Design review of the part built by this model. Coordinates are the model's own, in mm. Face numbers are marked on the shaded views. A direction names the side the tool comes from. Coordinates: 2 decimals unless noted, no trailing zeros. Loops run counter-clockwise (first coordinate to the right, second up) from the corner with the lowest first, then second, coordinate; pieces in that order, holes last. Notation, with made-up numbers: M -5.75,-33.75 L 7.25,-33.75 A13 cw 7.25,-21.75 Z; hole C -31.5,63.5 d11. An arc over 180 degrees is marked long. Put each result on its own line as item: value. Start each with the question number.
(1) Take a section at D-D, the plane y = 2.5. Give the boundary of the cut face in (x, z), then the cut area to 3 significant figures.
(2) For probe 1 along X at (y, z) = (-5.75, 3.25); probe 2 along X at (y, z) = (-0.75, 0.5); probe 3 along Z at (x, y) = (14.5, 0), list the stretches that pass through material, from the lowest coordinate up. Write a range as [from, to].
(3) Take a section at A-A, the plane x = 20. Count the separate pieces of the cut face and the enclosed holes in it, then the cut area to 3 significant figures.
(4) The part is to be moulded in two halves that separate along Y. For the marked faces 1, 2, 3 and 4, say which applies: +Y half, -Y half, draft (parallel to the pull), parting line (faces both ways), or undercut.
(5) For the marked faces 5, 6 and 7, list the 3-axis set-ups (+Z, -Z, +X, -X, +Y, -Y) from which the entire face can be reached by the end or side of a thin tool; tool diameter is ignored.
(6) Clearance check with flat-ended pins moving along their axes: pin 1 (8 mm diameter, centred on x = 23, y = -1.5, fed in from -Z); pin 2 (2 mm diameter, centred on x = 23, z = 1, fed in from -Y); pin 3 (1.3 mm diameter, centred on x = 14.5, z = 1.5, fed in from -Y); pin 4 (1 mm diameter, centred on x = 0.5, y = -3.5, fed in from +Z). State where each tip first meets the part, or that it passes through.
Autodesk Inventor part; units mm, degrees
ref_plane "YZ Plane" through (0, 0, 0) normal (1, 0, 0) x (0, 1, 0)
ref_plane "XZ Plane" through (0, 0, 0) normal (0, 1, 0) x (-1, 0, 0)
ref_plane "XY Plane" through (0, 0, 0) normal (0, 0, 1) x (1, 0, 0)
sketch "Sketch1" plane through (0, 0, 0) normal (0, 0, 1) x (1, 0, 0)
  line L0 (-21.147, 7.3925) -> (29.653, 7.3925)
  line L1 (29.653, 7.3925) -> (29.653, -5.3075)
  line L2 (29.653, -5.3075) -> (-21.147, -5.3075)
  line L3 (-21.147, -5.3075) -> (-21.147, 7.3925)
  point P0 (0, 0)
  dimension "d0" = 50.8
  dimension "d1" = 12.7
extrude "Extrusion1" add sketch "Sketch1" along normal blind 2.54
sketch "Sketch3" plane through (29.653, -5.3075, 0) normal (1, 0, 0) x (0, 0, -1)
  line L0 (-2.54, 0) -> (-8.89, 0)
  line L1 (-8.89, 0) -> (-8.89, -6.35)
  line L2 (-8.89, -6.35) -> (-2.54, -6.35)
  line L3 (-2.54, -6.35) -> (-2.54, 0)
  point P0 (0, 5.3075)
  dimension "d9" = 6.35
  dimension "d10" = 6.35
extrude "Extrusion2" add sketch "Sketch3" against normal blind 50.8
fillet "Fillet1" radius 3.175 3 edges at (4.253, -5.3075, 8.89) (4.253, -11.6575, 8.89) (4.253, -11.6575, 2.54)
hole "Hole1" at (29.653, -8.4825, 5.715) direction (-1, 0, 0) diameter 5.08 end through all
sketch "Sketch4" plane through (-21.147, -5.3075, 2.54) normal (0, 1, 0) x (1, 0, 0)
  line L0 (50.8, 0) -> (0, 0)
  line L1 (0, 0) -> (0, -3.175)
  line L2 (6.35, 0) -> (12.7, 0)
  line L3 (12.7, 0) -> (12.7, -6.6787)
  line L4 (12.7, -6.6787) -> (6.35, -6.6787)
  line L5 (6.35, -6.6787) -> (6.35, 0)
  line L6 (19.05, 0) -> (25.4, 0)
  line L7 (25.4, 0) -> (25.4, -6.6787)
  line L8 (25.4, -6.6787) -> (19.05, -6.6787)
  line L9 (19.05, -6.6787) -> (19.05, 0)
  line L10 (31.75, 0) -> (38.1, 0)
  line L11 (38.1, 0) -> (38.1, -6.6787)
  line L12 (38.1, -6.6787) -> (31.75, -6.6787)
  line L13 (31.75, -6.6787) -> (31.75, 0)
  point P0 (21.147, 2.54)
  dimension "d23" = 6.35
  dimension "d24" = 6.35
  dimension "d25" = 6.35
  dimension "d26" = 6.35
  dimension "d27" = 6.35
  dimension "d28" = 6.35
extrude "Extrusion3" cut sketch "Sketch4" against normal blind 12.7
hole "Hole2" at (-9.717, 1.0425, 2.54) direction (0, 0, -1) diameter 4.9784 end through all
hole "Hole3" at (18.223, 1.0425, 2.54) direction (0, 0, -1) diameter 4.9784 end through all
hole "Hole4" at (4.253, 1.0425, 2.54) direction (0, 0, -1) diameter 4.9784 end through all
sketch "Sketch5" plane through (29.653, -8.4825, 2.54) normal (0, 0, -1) x (-1, 0, 0)
  line L0 (12.7, 0) -> (12.7, 3.175)
  line L1 (0, 3.175) -> (12.7, 3.175)
  line L2 (0, 3.175) -> (12.7, 3.175)
  line L3 (12.7, 3.175) -> (12.7, 0)
  line L4 (12.7, 0) -> (0, 0)
  line L5 (0, 0) -> (0, 3.175)
  point P0 (29.653, 8.4825)
sketch "Sketch6" plane through (10.603, -8.4825, 2.54) normal (0, 0, -1) x (-1, 0, 0)
  line L0 (0, 3.175) -> (0, 0)
  line L1 (6.35, 0) -> (0, 0)
  line L2 (0, 3.175) -> (6.35, 3.175)
  line L3 (6.35, 3.175) -> (6.35, 0)
  line L4 (6.35, 0) -> (0, 0)
  line L5 (0, 0) -> (0, 3.175)
  point P0 (10.603, 8.4825)
sketch "Sketch7" plane through (-2.097, -8.4825, 2.54) normal (0, 0, -1) x (-1, 0, 0)
  line L0 (0, 3.175) -> (0, 0)
  line L1 (6.35, 0) -> (0, 0)
  line L2 (0, 3.175) -> (6.35, 3.175)
  line L3 (6.35, 3.175) -> (6.35, 0)
  line L4 (6.35, 0) -> (0, 0)
  line L5 (0, 0) -> (0, 3.175)
  point P0 (-2.097, 8.4825)
sketch "Sketch8" plane through (-21.147, -8.4825, 2.54) normal (0, 0, -1) x (-1, 0, 0)
  line L0 (-6.35, 3.175) -> (-6.35, 0)
  line L1 (0, 0) -> (-6.35, 0)
  line L2 (-6.35, 3.175) -> (0, 3.175)
  line L3 (0, 3.175) -> (0, 0)
  line L4 (0, 0) -> (-6.35, 0)
  line L5 (-6.35, 0) -> (-6.35, 3.175)
  point P0 (-21.147, 8.4825)
extrude "Extrusion4" add sketch "Sketch5" along normal blind 2.54
extrude "Extrusion5" add sketch "Sketch6" along normal blind 2.54
extrude "Extrusion6" add sketch "Sketch7" along normal blind 2.54
extrude "Extrusion7" add sketch "Sketch8" along normal blind 2.54
properties part number "HingeP1"
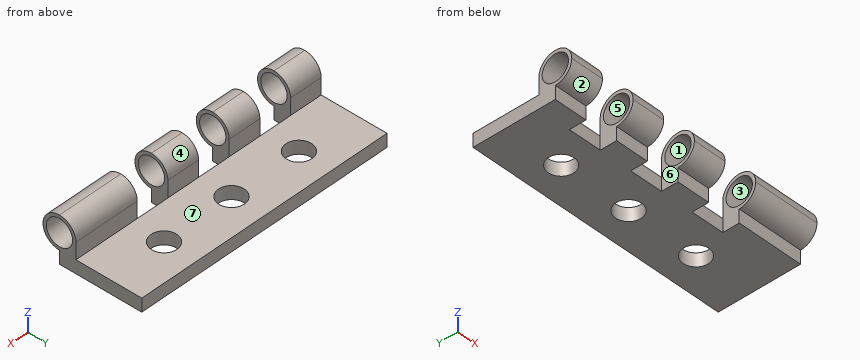
Computed values:
1. outline: M -21.15,0 L -11.73,0 L -11.73,2.54 L -21.15,2.54 Z; M -7.7,0 L 2.24,0 L 2.24,2.54 L -7.7,2.54 Z; M 6.27,0 L 16.21,0 L 16.21,2.54 L 6.27,2.54 Z; M 20.24,0 L 29.65,0 L 29.65,2.54 L 20.24,2.54 Z
1. area: 98.3 mm^2
2. probe 1: x = [-21.15, -14.8], [-8.45, -2.1], [4.25, 10.6], [16.95, 29.65]
2. probe 2: x = [-21.15, -11.44], [-7.99, 2.53], [5.98, 16.5], [19.95, 29.65]
2. probe 3: z = [0, 2.54]
3. separate pieces: 2
3. enclosed holes: 1
3. area: 45.0 mm^2
4. face 1: undercut
4. face 2: -Y half
4. face 3: undercut
4. face 4: +Y half
5. face 5: +X, -X
5. face 6: +Z, -Z, -Y
5. face 7: +Z, +X, -X, +Y
6. pin 1: stops at z = 0
6. pin 2: stops at y = -8.48
6. pin 3: stops at y = -5.31
6. pin 4: stops at z = 2.54
